The model under review builds one solid part; all positions refer to its coordinate system, in mm. Face numbers are marked on the shaded views. A direction names the side the tool comes from. Round coordinates to 2 decimals unless told otherwise and drop trailing zeros. Write each loop counter-clockwise with the first axis right and the second up, starting at its lowest first coordinate (ties: lowest second). Pieces come first, ordered by that corner, then holes. Notation, with made-up numbers: (35.5, -2.75) - (78.5, -2.75) arc R17 ccw to (78.5, 1.25) - close; hole circle Ø3 at (43, -21). An arc over 180 degrees is marked (long way). Return JSON: item names as keys, results as strings.
from build123d import *

# Parameters (mm, degrees)
SKETCH_1_R      = 1.35
EXTRUDE_2_DEPTH = 1.5
FILLET_1_R      = 0.5


with BuildPart() as part:
    # 草图1 → 凸台-拉伸2 (new body)
    with BuildSketch(Plane.XY):
        with BuildLine():
            Line((97.519773553, 11.5), (86.228033822, 11.5))
            ThreePointArc((86.228033822, 11.5), (85.16737365, 11.060660172), (84.728033822, 10))
            Line((84.728033822, 10), (84.728033822, 7))
            Line((84.728033822, 7), (84.728033822, -3))
            Line((84.728033822, -3), (84.728033822, -6))
            ThreePointArc((84.728033822, -6), (85.16737365, -7.060660172), (86.228033822, -7.5))
            Line((86.228033822, -7.5), (97.519773553, -7.5))
            ThreePointArc((97.519773553, -7.5), (98.580433725, -7.060660172), (99.019773553, -6))
            Line((99.019773553, -6), (99.019773553, -3))
            Line((99.019773553, -3), (99.019773553, 7))
            Line((99.019773553, 7), (99.019773553, 10))
            ThreePointArc((99.019773553, 10), (98.580433725, 11.060660172), (97.519773553, 11.5))
        make_face()
        with Locations((87.478033822, -4.75)):
            Circle(SKETCH_1_R, mode=Mode.SUBTRACT)
        with Locations((96.269773553, -4.75)):
            Circle(SKETCH_1_R, mode=Mode.SUBTRACT)
        with Locations((96.269773553, 8.75)):
            Circle(SKETCH_1_R, mode=Mode.SUBTRACT)
        with Locations((87.478033822, 8.75)):
            Circle(SKETCH_1_R, mode=Mode.SUBTRACT)
        with BuildLine():
            Line((88.728033822, 5.5), (95.019773553, 5.5))
            ThreePointArc((95.019773553, 5.5), (95.726880334, 5.207106781), (96.019773553, 4.5))
            Line((96.019773553, 4.5), (96.019773553, -0.5))
            ThreePointArc((96.019773553, -0.5), (95.726880334, -1.207106781), (95.019773553, -1.5))
            Line((95.019773553, -1.5), (88.728033822, -1.5))
            ThreePointArc((88.728033822, -1.5), (88.020927041, -1.207106781), (87.728033822, -0.5))
            Line((87.728033822, -0.5), (87.728033822, 4.5))
            ThreePointArc((87.728033822, 4.5), (88.020927041, 5.207106781), (88.728033822, 5.5))
        make_face(mode=Mode.SUBTRACT)
    extrude(amount=EXTRUDE_2_DEPTH)

    # 圆角1
    fillet_1_edges = [part.edges().sort_by_distance(p)[0] for p in [
        (85.16737365, 11.060660172, 1.5),
        (84.728033822, 2, 1.5),
        (85.16737365, -7.060660172, 1.5),
        (91.873903688, -7.5, 1.5),
        (98.580433725, -7.060660172, 1.5),
        (99.019773553, 2, 1.5),
        (98.580433725, 11.060660172, 1.5),
        (91.873903688, 11.5, 1.5),
    ]]
    fillet(fillet_1_edges, radius=FILLET_1_R)


solid = part.part
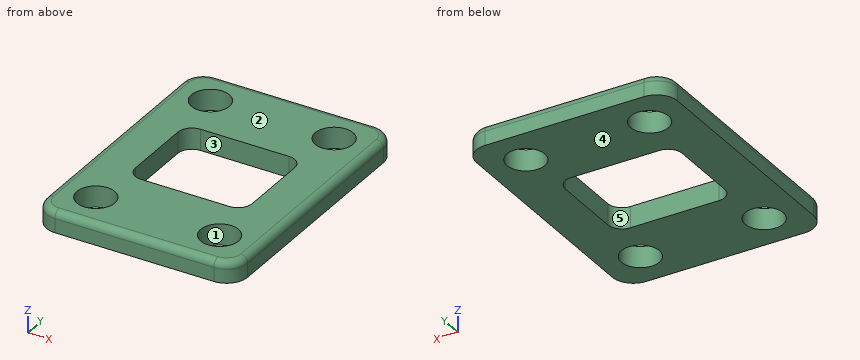
(1) Add section C-C (z = 0.5). Write out the cut boundary in (x, y), plus the area to 3 significant figures.
Filled in:
{"outline": "(84.73, -6) arc R1.5 ccw to (86.23, -7.5) - (97.52, -7.5) arc R1.5 ccw to (99.02, -6) - (99.02, 10) arc R1.5 ccw to (97.52, 11.5) - (86.23, 11.5) arc R1.5 ccw to (84.73, 10) - close; hole circle Ø2.7 at (87.48, -4.75); hole circle Ø2.7 at (87.48, 8.75); hole (87.73, -0.5) arc R1 ccw to (88.73, -1.5) - (95.02, -1.5) arc R1 ccw to (96.02, -0.5) - (96.02, 4.5) arc R1 ccw to (95.02, 5.5) - (88.73, 5.5) arc R1 ccw to (87.73, 4.5) - close; hole circle Ø2.7 at (96.27, -4.75); hole circle Ø2.7 at (96.27, 8.75)", "area": "190 mm2"}
(2) Add section D-D (y = 8.75). Write out the cut boundary in (x, z).
Filled in:
{"outline": "(84.73, 0) - (86.13, 0) - (86.13, 1.5) - (85.23, 1.5) arc R0.5 ccw to (84.73, 1) - close; (88.83, 0) - (94.92, 0) - (94.92, 1.5) - (88.83, 1.5) - close; (97.62, 0) - (99.02, 0) - (99.02, 1) arc R0.5 ccw to (98.52, 1.5) - (97.62, 1.5) - close"}
(3) Add section B-B (x = 91). Write out the cut boundary in (y, z), plus the area to 3 significant figures.
Filled in:
{"outline": "(-7.5, 0) - (-1.5, 0) - (-1.5, 1.5) - (-7, 1.5) arc R0.5 ccw to (-7.5, 1) - close; (5.5, 0) - (11.5, 0) - (11.5, 1) arc R0.5 ccw to (11, 1.5) - (5.5, 1.5) - close", "area": "17.9 mm2"}
(4) For the marked faces 4 and 5, list the 3-axis set-ups (+Z, -Z, +X, -X, +Y, -Y) from which the entire face can be reached by the end or side of a thin tool; tool diameter is ignored.
Filled in:
{"face 4": "-Z, +X, -X, +Y, -Y", "face 5": "+Z, -Z"}
(5) Wall thickness on line 1 (Y direction, x = 91.5, z = 1); line 2 (X direction, y = 9, z = 0.85); line 3 (Y direction, x = 87, z = 0.8): over which ranges is each line inside the solid? List them lowest first.
Filled in:
{"line 1": "y = -7.5 to -1.5, 5.5 to 11.5", "line 2": "x = 84.73 to 86.15, 88.8 to 94.94, 97.6 to 99.02", "line 3": "y = -7.5 to -6.01, -3.49 to 7.49, 10.01 to 11.5"}
(6) Mouldability with a two-part tool opening along Y and no side actions: class the marked faces 1, 2 and 3 as released by +Y, released by -Y, zero draft, split by the parting line, or undercut.
Filled in:
{"face 1": "undercut", "face 2": "zero draft", "face 3": "undercut"}
(7) Clearance check with a flat-ended pin moving along its axis: pin 1 Ø3.5 at (x, y) = (87.48, -4.75) entering from -Z. State where the tip first meets the part, or that it passes through.
Filled in:
{"pin 1": "stops at z = 0"}
(8) Add section A-A (y = -0.25). Write out the cut boundary in (x, z), plus the area to 3 significant figures.
Filled in:
{"outline": "(84.73, 0) - (87.73, 0) - (87.73, 1.5) - (85.23, 1.5) arc R0.5 ccw to (84.73, 1) - close; (96.02, 0) - (99.02, 0) - (99.02, 1) arc R0.5 ccw to (98.52, 1.5) - (96.02, 1.5) - close", "area": "8.89 mm2"}
